Read the model definition and answer for the solid it produces. Units are mm, in the model's axes. Coordinates: 2 decimals unless noted, no trailing zeros. Order: outer loops, then holes, each group sorted by start corner. A loop starts at its lowest first (then second) coordinate and runs counter-clockwise, first axis right, second up. Notation, with made-up numbers: (27.5, -15.5) - (64.5, -15.5) arc R22 cw to (64.5, 11.5) - close; hole circle Ø6 at (31.5, -30). An arc over 180 degrees is marked (long way). Write item = value, one per line.
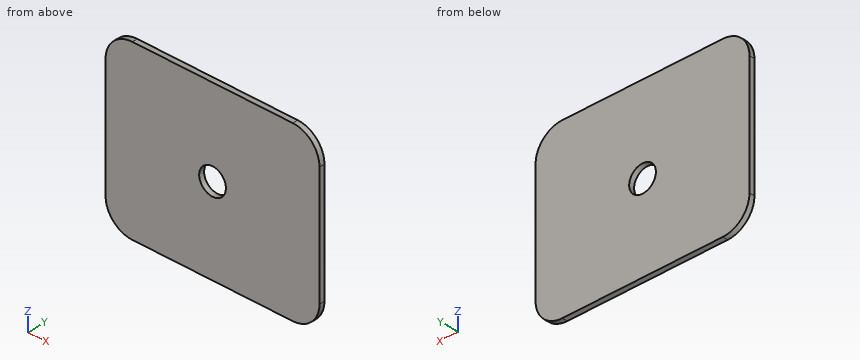
from build123d import *

# Parameters (mm, degrees)
SKETCH_10_R     = 5
EXTRUDE_1_DEPTH = 2


with BuildPart() as part:
    # Эскиз10 → Вытянуть1 (new body)
    with BuildSketch(Plane(origin=(0, 0, 0), x_dir=(1, 0, 0), z_dir=(0, 1, 0))):
        with BuildLine():
            Line((-30, 2), (30, 2))
            ThreePointArc((30, 2), (37.071067812, -0.928932188), (40, -8))
            Line((40, -8), (40, -53))
            ThreePointArc((40, -53), (37.071067812, -60.071067812), (30, -63))
            Line((30, -63), (-30, -63))
            ThreePointArc((-30, -63), (-37.071067812, -60.071067812), (-40, -53))
            Line((-40, -53), (-40, -8))
            ThreePointArc((-40, -8), (-37.071067812, -0.928932188), (-30, 2))
        make_face()
        with Locations(Location((0, -30.5, 0), (0, 0, 270))):
            Circle(SKETCH_10_R, mode=Mode.SUBTRACT)
    extrude(amount=EXTRUDE_1_DEPTH)


solid = part.part
1) The part is cut by section A-A (x = 0). Determine the outline of the cut face in (y, z).
Returned:
outline = (0, -2) - (2, -2) - (2, 25.5) - (0, 25.5) - close; (0, 35.5) - (2, 35.5) - (2, 63) - (0, 63) - close
2) Straight lines are drawn through the part: line 1 along X through (y, z) = (0.6, 30.5); line 2 along X through (y, z) = (1.65, 5); line 3 along X through (y, z) = (1.25, 54). For each, find the intervals that lie inside material, in ascending order. Write a range as from..to.
Returned:
line_1 = -40..-5, 5..40
line_2 = -39.54..39.54
line_3 = -39.95..39.95
3) The part is cut by section C-C (z = 30.5). Determine the outline of the cut face in (x, y), and give its area (3 significant figures).
Returned:
outline = (-40, 0) - (-5, 0) - (-5, 2) - (-40, 2) - close; (5, 0) - (40, 0) - (40, 2) - (5, 2) - close
area = 140 mm^2
4) The part is cut by section B-B (y = 0.35). Determine the outline of the cut face in (x, z).
Returned:
outline = (-40, 8) arc R10 ccw to (-30, -2) - (30, -2) arc R10 ccw to (40, 8) - (40, 53) arc R10 ccw to (30, 63) - (-30, 63) arc R10 ccw to (-40, 53) - close; hole circle Ø10 at (0, 30.5)
